Source: CAD feature listing. Evaluate the final solid. Frame: model axes, mm. Coordinates: 2 decimals unless noted, no trailing zeros. Order: outer loops, then holes, each group sorted by start corner. A loop starts at its lowest first (then second) coordinate and runs counter-clockwise, first axis right, second up. Notation, with made-up numbers: (26.5, 33) - (67.5, 33) arc R17 ccw to (67.5, 58) - close; hole circle Ø11 at (-34.75, 2.5). An arc over 180 degrees is marked (long way). One line per question, with ' | ' between items. Start each with the question number.
(1) Section A-A (z = 225.5). Return the cut outline in (x, y).
(2) Draft query along Y for faces 1 (the flat face through (-81, 316, 750)), 2 (the flat face through (-81.347, 314.859, 380.25)), 3 (the flat face through (-81.96, 315.8, 380.25)). Return one class per face: +Y half, -Y half, draft (parallel to the pull), parting line (faces both ways), or undercut.
(3) Contact query for flat-ended pins moving along their axis: P1, Ø4, axis at x = -95, z = 108.5, coming from the +Y side; P2, Ø1, axis at x = -78.5, z = 328, coming from the -Y side; P3, Ø1, axis at y = 313, z = 444, coming from the +X side. Output: stop coordinate, or through.
(4) Line query: line 1 along X through (y, z) = (298.65, 495); line 2 along Z through (x, y) = (-86, 308.5); line 3 along X through (y, z) = (298.5, 495). Output: solid intervals per line, ascending.
from build123d import *

# Parameters (mm, degrees)
SKETCH2_W           = 7.85
SKETCH2_H           = 1
BOSS_EXTRUDE2_DEPTH = 750
EDGE_FLANGE9_DEPTH  = 750
EDGE_FLANGE10_DEPTH = 750
SKETCH57_R          = 1.6
CUT_EXTRUDE2_DEPTH  = 10
SKETCH58_R          = 1.6
CUT_EXTRUDE3_DEPTH  = 10
SKETCH59_R          = 1.6
CUT_EXTRUDE4_DEPTH  = 10
SKETCH60_R          = 1.6
CUT_EXTRUDE5_DEPTH  = 3
CUT_EXTRUDE6_DEPTH  = 3
CUT_EXTRUDE7_DEPTH  = 10
SKETCH63_R          = 1.6
CUT_EXTRUDE8_DEPTH  = 10


# Sheet-metal steps are written as plain solids
with BuildPart() as part:
    # Sketch2 → Boss-Extrude2 (new body)
    with BuildSketch(Plane.XY):
        with Locations((-96.082096866, 298.73456983)):
            Rectangle(SKETCH2_W, SKETCH2_H)
    extrude(amount=BOSS_EXTRUDE2_DEPTH)

    # Edge-Flange9 section (across the edge) → Edge-Flange9 (add)
    with BuildSketch(Plane(origin=(-91.52201157, 299.23456983, 750), x_dir=(-0.8660254037844364, 0.5000000000000041, 0), z_dir=(0, 0, -1))):
        with BuildLine():
            Line((-1, 0.635085296), (-1, 37.112649731))
            Line((-1, 37.112649731), (0, 37.112649731))
            Line((0, 37.112649731), (0, 0.635085296))
            ThreePointArc((0, 0.635085296), (0.147372056, 0.085085296), (0.55, -0.317542648))
            Line((0.55, -0.317542648), (0.05, -1.183568052))
            ThreePointArc((0.05, -1.183568052), (-0.718653348, -0.414914704), (-1, 0.635085296))
        make_face()
    extrude(amount=EDGE_FLANGE9_DEPTH)

    # Edge-Flange10 section (across the edge) → Edge-Flange10 (add)
    with BuildSketch(Plane(origin=(-72.648144057, 331.925067298, 750), x_dir=(-0.8660254037844433, -0.49999999999999195, 0), z_dir=(0, 0, -1))):
        with BuildLine():
            Line((-1, 0.635085296), (-1, 8.49))
            Line((-1, 8.49), (0, 8.49))
            Line((0, 8.49), (0, 0.635085296))
            ThreePointArc((0, 0.635085296), (0.147372056, 0.085085296), (0.55, -0.317542648))
            Line((0.55, -0.317542648), (0.05, -1.183568052))
            ThreePointArc((0.05, -1.183568052), (-0.718653348, -0.414914704), (-1, 0.635085296))
        make_face()
    extrude(amount=EDGE_FLANGE10_DEPTH)

    # Sketch57 → Cut-Extrude2 (cut)
    with BuildSketch(Plane.XZ.offset(-298.23456983)):
        with Locations(Location((-96.082096866, 735, 0), (0, 0, 270))):
            Circle(SKETCH57_R)
        with Locations(Location((-96.082096866, 15, 0), (0, 0, 270))):
            Circle(SKETCH57_R)
        with Locations(Location((-96.082096866, 75, 0), (0, 0, 270))):
            Circle(SKETCH57_R)
        with Locations(Location((-96.082096866, 135, 0), (0, 0, 270))):
            Circle(SKETCH57_R)
        with Locations(Location((-96.082096866, 195, 0), (0, 0, 270))):
            Circle(SKETCH57_R)
        with Locations(Location((-96.082096866, 255, 0), (0, 0, 270))):
            Circle(SKETCH57_R)
        with Locations(Location((-96.082096866, 315, 0), (0, 0, 270))):
            Circle(SKETCH57_R)
        with Locations(Location((-96.082096866, 375, 0), (0, 0, 270))):
            Circle(SKETCH57_R)
        with Locations(Location((-96.082096866, 435, 0), (0, 0, 270))):
            Circle(SKETCH57_R)
        with Locations(Location((-96.082096866, 495, 0), (0, 0, 270))):
            Circle(SKETCH57_R)
        with Locations(Location((-96.082096866, 555, 0), (0, 0, 270))):
            Circle(SKETCH57_R)
        with Locations(Location((-96.082096866, 615, 0), (0, 0, 270))):
            Circle(SKETCH57_R)
        with Locations(Location((-96.082096866, 675, 0), (0, 0, 270))):
            Circle(SKETCH57_R)
    extrude(amount=-CUT_EXTRUDE2_DEPTH, mode=Mode.SUBTRACT)

    # Sketch58 → Cut-Extrude3 (cut)
    with BuildSketch(Plane(origin=(90.107687578, 52.023697679, 0), x_dir=(0, 0, -1), z_dir=(0.8660254037844434, 0.4999999999999918, 0))):
        with Locations(Location((-735, 328.34215511, 0), (0, 0, 90))):
            Circle(SKETCH58_R)
        with Locations(Location((-15, 328.34215511, 0), (0, 0, 90))):
            Circle(SKETCH58_R)
        with Locations(Location((-75, 328.34215511, 0), (0, 0, 90))):
            Circle(SKETCH58_R)
        with Locations(Location((-135, 328.34215511, 0), (0, 0, 90))):
            Circle(SKETCH58_R)
        with Locations(Location((-195, 328.34215511, 0), (0, 0, 90))):
            Circle(SKETCH58_R)
        with Locations(Location((-255, 328.34215511, 0), (0, 0, 90))):
            Circle(SKETCH58_R)
        with Locations(Location((-315, 328.34215511, 0), (0, 0, 90))):
            Circle(SKETCH58_R)
        with Locations(Location((-375, 328.34215511, 0), (0, 0, 90))):
            Circle(SKETCH58_R)
        with Locations(Location((-435, 328.34215511, 0), (0, 0, 90))):
            Circle(SKETCH58_R)
        with Locations(Location((-495, 328.34215511, 0), (0, 0, 90))):
            Circle(SKETCH58_R)
        with Locations(Location((-555, 328.34215511, 0), (0, 0, 90))):
            Circle(SKETCH58_R)
        with Locations(Location((-615, 328.34215511, 0), (0, 0, 90))):
            Circle(SKETCH58_R)
        with Locations(Location((-675, 328.34215511, 0), (0, 0, 90))):
            Circle(SKETCH58_R)
    extrude(amount=-CUT_EXTRUDE3_DEPTH, mode=Mode.SUBTRACT)

    # Sketch59 → Cut-Extrude4 (cut)
    with BuildSketch(Plane(origin=(-198.213878259, 114.43883597, 0), x_dir=(0, 0, 1), z_dir=(-0.8660254037844364, 0.5000000000000041, 0))):
        with Locations(Location((35, 232.257600891, 0), (0, 0, 270))):
            Circle(SKETCH59_R)
        with Locations(Location((60, 232.257600891, 0), (0, 0, 270))):
            Circle(SKETCH59_R)
        with Locations(Location((85, 232.257600891, 0), (0, 0, 270))):
            Circle(SKETCH59_R)
        with Locations(Location((110, 232.257600891, 0), (0, 0, 270))):
            Circle(SKETCH59_R)
        with Locations(Location((135, 232.257600891, 0), (0, 0, 270))):
            Circle(SKETCH59_R)
        with Locations(Location((160, 232.257600891, 0), (0, 0, 270))):
            Circle(SKETCH59_R)
        with Locations(Location((185, 232.257600891, 0), (0, 0, 270))):
            Circle(SKETCH59_R)
        with Locations(Location((210, 232.257600891, 0), (0, 0, 270))):
            Circle(SKETCH59_R)
        with Locations(Location((235, 232.257600891, 0), (0, 0, 270))):
            Circle(SKETCH59_R)
        with Locations(Location((260, 232.257600891, 0), (0, 0, 270))):
            Circle(SKETCH59_R)
        with Locations(Location((285, 232.257600891, 0), (0, 0, 270))):
            Circle(SKETCH59_R)
        with Locations(Location((310, 232.257600891, 0), (0, 0, 270))):
            Circle(SKETCH59_R)
        with Locations(Location((335, 232.257600891, 0), (0, 0, 270))):
            Circle(SKETCH59_R)
        with Locations(Location((360, 232.257600891, 0), (0, 0, 270))):
            Circle(SKETCH59_R)
        with Locations(Location((385, 232.257600891, 0), (0, 0, 270))):
            Circle(SKETCH59_R)
        with Locations(Location((410, 232.257600891, 0), (0, 0, 270))):
            Circle(SKETCH59_R)
        with Locations(Location((435, 232.257600891, 0), (0, 0, 270))):
            Circle(SKETCH59_R)
        with Locations(Location((460, 232.257600891, 0), (0, 0, 270))):
            Circle(SKETCH59_R)
        with Locations(Location((485, 232.257600891, 0), (0, 0, 270))):
            Circle(SKETCH59_R)
        with Locations(Location((510, 232.257600891, 0), (0, 0, 270))):
            Circle(SKETCH59_R)
    extrude(amount=-CUT_EXTRUDE4_DEPTH, mode=Mode.SUBTRACT)

    # Sketch60 → Cut-Extrude5 (cut)
    with BuildSketch(Plane(origin=(-198.213878259, 114.43883597, 0), x_dir=(0, 0, 1), z_dir=(-0.8660254037844364, 0.5000000000000041, 0))):
        with Locations(Location((26.5, 248.107600891, 0), (0, 0, 270))):
            Circle(SKETCH60_R)
        with Locations(Location((26.5, 216.407600891, 0), (0, 0, 270))):
            Circle(SKETCH60_R)
    extrude(amount=-CUT_EXTRUDE5_DEPTH, mode=Mode.SUBTRACT)

    # Sketch61 → Cut-Extrude6 (cut)
    with BuildSketch(Plane(origin=(-198.213878259, 114.43883597, 0), x_dir=(0, 0, 1), z_dir=(-0.8660254037844364, 0.5000000000000041, 0))):
        with BuildLine():
            Line((21.25, 236.757600891), (21.25, 227.757600891))
            ThreePointArc((21.25, 227.757600891), (21.103553391, 227.404047501), (20.75, 227.257600891))
            Line((20.75, 227.257600891), (18.75, 227.257600891))
            ThreePointArc((18.75, 227.257600891), (18.396446609, 227.404047501), (18.25, 227.757600891))
            Line((18.25, 227.757600891), (18.25, 236.757600891))
            ThreePointArc((18.25, 236.757600891), (18.396446609, 237.111154282), (18.75, 237.257600891))
            Line((18.75, 237.257600891), (20.75, 237.257600891))
            ThreePointArc((20.75, 237.257600891), (21.103553391, 237.111154282), (21.25, 236.757600891))
        make_face()
    extrude(amount=-CUT_EXTRUDE6_DEPTH, mode=Mode.SUBTRACT)

    # Sketch62 → Cut-Extrude7 (cut)
    with BuildSketch(Plane(origin=(-198.213878259, 114.43883597, 0), x_dir=(0, 0, 1), z_dir=(-0.8660254037844364, 0.5000000000000041, 0))):
        with BuildLine():
            Line((729, 239.257600891), (729, 225.257600891))
            ThreePointArc((729, 225.257600891), (725, 221.257600891), (721, 225.257600891))
            Line((721, 225.257600891), (721, 239.257600891))
            ThreePointArc((721, 239.257600891), (725, 243.257600891), (729, 239.257600891))
        make_face()
    extrude(amount=-CUT_EXTRUDE7_DEPTH, mode=Mode.SUBTRACT)

    # Sketch63 → Cut-Extrude8 (cut)
    with BuildSketch(Plane(origin=(-198.213878259, 114.43883597, 0), x_dir=(0, 0, 1), z_dir=(-0.8660254037844364, 0.5000000000000041, 0))):
        with Locations(Location((8, 232.257600891, 0), (0, 0, 270))):
            Circle(SKETCH63_R)
        with Locations(Location((638, 232.257600891, 0), (0, 0, 270))):
            Circle(SKETCH63_R)
        with Locations(Location((742, 232.257600891, 0), (0, 0, 270))):
            Circle(SKETCH63_R)
    extrude(amount=-CUT_EXTRUDE8_DEPTH, mode=Mode.SUBTRACT)


solid = part.part
Response values:
1) outline: (-100.01, 298.23) - (-92.16, 298.23) arc R2.1 ccw to (-90.34, 299.28) - (-72.1, 330.88) arc R2.1 ccw to (-72.1, 332.98) - (-76.03, 339.78) - (-76.89, 339.28) - (-72.97, 332.48) arc R1.1 cw to (-72.97, 331.38) - (-91.2, 299.78) arc R1.1 cw to (-92.16, 299.23) - (-100.01, 299.23) - close
2) face 1: draft | face 2: -Y half | face 3: undercut
3) P1: stops at y = 299.23 | P2: stops at y = 318.92 | P3: stops at x = -82.13
4) line 1: x = -100.01 to -97.68, -94.48 to -90.9 | line 2: z = 0 to 721.15, 728.85 to 750 | line 3: x = -100.01 to -97.68, -94.48 to -91.14
